Autodesk Inventor part; units mm, degrees
ref_plane "YZ Plane" through (0, 0, 0) normal (1, 0, 0) x (0, 1, 0)
ref_plane "XZ Plane" through (0, 0, 0) normal (0, 1, 0) x (-1, 0, 0)
ref_plane "XY Plane" through (0, 0, 0) normal (0, 0, 1) x (1, 0, 0)
sketch "Sketch1" plane through (0, 0, 0) normal (1, 0, 0) x (0, 1, 0)
  line L0 (0, 0) -> (-9.28, 0)
  line L1 (0, 0) -> (0, 2)
  line L2 (0, 2) -> (12, 2)
  line L3 (12, 2) -> (12, 7)
  line L4 (12, 7) -> (14, 7)
  line L5 (14, 7) -> (14, 11)
  line L6 (14, 11) -> (35.7, 11)
  line L7 (35.7, 11) -> (35.7, 10.25)
  line L8 (35.7, 10.25) -> (68, 10.25)
  line L9 (68, 10.25) -> (68, 0)
  line L10 (68, 0) -> (0, 0)
  dimension "d0" = 4
  dimension "d2" = 12
  dimension "d3" = 2
  dimension "d5" = 22
  dimension "d6" = 20.5
  dimension "d7" = 32.3
  dimension "d8" = 21.7
  dimension "d32" = 14
revolve "Revolution1" add sketch "Sketch1" angle 360 about axis through (0, 0, 0) along (0, -1, 0)
sketch "Sketch2" plane through (0, 14, 0) normal (0, -1, 0) x (1, 0, 0)
  circle A0 centre (0, 0) radius 11
  point P0 (0, 9)
  point P1 (-9, 0)
  point P2 (0, -9)
  point P3 (9, 0)
  dimension "d12" = 360
  dimension "d15" = 18
hole "Hole1" at (0, 14, 9) at (-9, 14, 0) at (0, 14, -9) at (9, 14, 0) direction (0, 1, 0) diameter 1.567 depth 4 tip angle 118
sketch "Sketch3" plane through (0, 12, 0) normal (0, -1, 0) x (1, 0, 0)
  circle A0 centre (0, 0) radius 7
  circle A1 centre (0, 0) radius 2
  line L0 (1.6931, 6.7922) -> (6.7922, 1.6931)
  line L1 (-1.6931, -6.7922) -> (-6.7922, -1.6931)
  line L2 (0, 0) -> (-24.8191, 0) construction
  dimension "d23" = 135
  dimension "d24" = 12
extrude "Extrusion1" cut sketch "Sketch3" against normal up to surface (2 mm away) contours L0 A0 | A0 L1
sketch "Sketch4" plane through (0, 0, 0) normal (0, -1, 0) x (1, 0, 0)
  circle A0 centre (0, 0) radius 2
  line L0 (1.5, 1.3229) -> (1.5, -1.3229)
  dimension "d28" = 1.5
extrude "Extrusion2" cut sketch "Sketch4" against normal blind 8 contours A0 L0 picked at (1.5908, -0.3089)
sketch "Sketch5" plane through (0, 68, 0) normal (0, 1, 0) x (1, 0, 0)
  circle A0 centre (0, 0) radius 10.25
  line L0 (-6.7082, 7.75) -> (6.7082, 7.75)
  line L1 (6.7082, -7.75) -> (-6.7082, -7.75)
  dimension "d33" = 15.5
extrude "Extrusion3" cut sketch "Sketch5" against normal up to surface (32.3 mm away) contours L0 A0 | A0 L1
properties part number "Motor"
Could you check a few things on this model? Use its own coordinates, in mm. A direction names the side the tool comes from. Give positions to 0.01 mm unless a question says otherwise; leave off trailing zeros. Order: outer loops, then holes, each group sorted by start corner. A loop starts at its lowest first (then second) coordinate and runs counter-clockwise, first axis right, second up. Notation, with made-up numbers: (55.25, 56) -> (114.25, 56) arc R21 ccw to (114.25, 67) -> close; hole circle Ø5 at (-9.75, 26.5). An arc over 180 degrees is marked (long way). Answer in a Markdown table with one row per item. Add a question column.
Item 1: We'd pull the mould along X, two halves only. Please class faces 1 (the flat face through (4.207, 12.986, 4.278)), 2 (the cylindrical face through (-2, 6, 0)), 3 (the conical face through (0.006, 18.389, 9.136)), 4 (the cylindrical face through (-0.235, 16.028, -9.747)): pulls with the +X half, pulls with the -X half, needs draft (parallel to the pull), parting line crosses it, or undercut.
Item 2: Imagine slicing it at A-A (z = -3.5). List the corners of the cut face in (x, y) for me, and give its area (3 significant figures).
Item 3: I'm going to push flat-ended pins straight in: P1, Ø5, axis at y = 19.5, z = 8.5, coming from the -X side; P2, Ø1, axis at y = 45, z = -5.5, coming from the -X side; P3, Ø2, axis at x = 0, z = 9, coming from the -Y side; P4, Ø7, axis at x = -3, z = 2.5, coming from the -Y side. Where does each tip first touch, or does it pass through?
Item 4: Imagine slicing it at C-C (y = 35). List the corners of the cut face in (x, z) for me.
Item 5: Please list where these lines run through material, in increasing order: probe 1 along X at (y, z) = (15.55, 0); probe 2 along Y at (x, z) = (1, 3.75).
Item 6: Imagine slicing it at B-B (y = 45.5). List the corners of the cut face in (x, z) for me, and give its area (3 significant figures).
Item 7: For faces 5 (the cylindrical face through (-8.235, 16.028, 0.17)), 6 (the flat face through (0, 52, -7.75)), 7 (the flat face through (0, 35.7, 8)), which set-ups out of +Z, -Z, +X, -X, +Y, -Y let a thin tool reach every point of the face, with its end or its side?
Item 8: Imagine slicing it at D-D (z = 5.75). List the corners of the cut face in (x, y) for me.
Result:
| question | item | result |
|---|---|---|
| 1 | face 1 | pulls with the +X half |
| 1 | face 2 | parting line crosses it |
| 1 | face 3 | undercut |
| 1 | face 4 | undercut |
| 2 | outline | (-10.43, 14) -> (-4.99, 14) -> (-4.99, 12) -> (6.06, 12) -> (6.06, 14) -> (10.43, 14) -> (10.43, 35.7) -> (9.63, 35.7) -> (9.63, 68) -> (-9.63, 68) -> (-9.63, 35.7) -> (-10.43, 35.7) -> close |
| 2 | area | 1,100 mm2 |
| 3 | P1 | x = -9.22 |
| 3 | P2 | x = -8.95 |
| 3 | P3 | y = 14 |
| 3 | P4 | y = 0 |
| 4 | outline | circle Ø22 at (0, 0) |
| 5 | probe 1 | -11 to -9.78, -8.22 to 8.22, 9.78 to 11 |
| 5 | probe 2 | 12 to 68 |
| 6 | outline | (-6.71, -7.75) -> (6.71, -7.75) arc R10.25 ccw to (6.71, 7.75) -> (-6.71, 7.75) arc R10.25 ccw to start |
| 6 | area | 284 mm2 |
| 7 | face 5 | -Y |
| 7 | face 6 | -Z, +X, -X, +Y |
| 7 | face 7 | +Y |
| 8 | outline | (-9.38, 14) -> (-3.99, 14) -> (-3.99, 12) -> (2.74, 12) -> (2.74, 14) -> (9.38, 14) -> (9.38, 35.7) -> (8.49, 35.7) -> (8.49, 68) -> (-8.49, 68) -> (-8.49, 35.7) -> (-9.38, 35.7) -> close |
